Input: part model. Units: mm. Frame: model coordinates. Round coordinates to 2 decimals unless told otherwise and drop trailing zeros. Loops run counter-clockwise (first coordinate to the right, second up) from the corner with the lowest first, then second, coordinate; pieces in that order, holes last. Notation, with made-up numbers: (26.25, -16.5) - (62.25, -16.5) arc R32 cw to (62.25, 9.5) - close; hole circle Ø11 at (17.25, 4). An arc over 180 degrees is marked (long way). One line per question, with ' | ' between items. Start each with the question number.
Item 1: Section C-C, the plane z = 3.25. Return loops of the section in (x, y).
Item 2: Section B-B, the plane x = 10.25. Return loops of the section in (y, z).
Item 3: First-contact query: pin 1 (0.7 mm diameter, centred on y = 6.5, z = 4, fed in from +X); pin 2 (0.5 mm diameter, centred on x = 6.5, y = 5, fed in from +Z); pin 3 (0.5 mm diameter, centred on x = 14, y = 6.5, fed in from -Z). Flat tips, straight axial feed; report the tip coordinate or a pass-through.
Item 4: Section A-A, the plane y = 4.5. Give the number of separate pieces and of enclosed holes in the cut face, plus the area to 3 significant figures.
Item 5: Draft query along X for faces 1 (the face through (10, 1, 0)), 2 (the face through (0, 1, 3)), 3 (the face through (10, 2.5, 2)), 4 (the face through (20, 1, 3)). Return one class per face: pulls with the +X half, pulls with the -X half, needs draft (parallel to the pull), parting line crosses it, or undercut.
Item 6: Material intervals for line 1 along Z through (x, y) = (14, 5); line 2 along Y through (x, z) = (4.75, 3.5); line 3 along X through (y, z) = (1.75, 4.65), sorted ascending.
```python
from build123d import *

# Parameters (mm, degrees)
ESQUISSE1_W        = 20
ESQUISSE1_H        = 5
BOSS_EXTRU_1_DEPTH = 2.5
ESQUISSE2_W        = 0.6
ESQUISSE2_H        = 0.6
BOSS_EXTRU_2_DEPTH = 6
CHANFREIN1_SIZE    = 0.1
CHANFREIN2_SIZE    = 0.5


with BuildPart() as part:
    # Esquisse1 → Boss.-Extru.1 (new body)
    with BuildSketch(Plane(origin=(0, 0, 0), x_dir=(1, 0, 0), z_dir=(0, 1, 0))):
        with Locations((10, -2.5)):
            Rectangle(ESQUISSE1_W, ESQUISSE1_H)
    extrude(amount=BOSS_EXTRU_1_DEPTH)

    # Esquisse2 → Boss.-Extru.2 (add)
    with BuildSketch(Plane(origin=(0, 2.5, 0), x_dir=(1, 0, 0), z_dir=(0, 1, 0))):
        with Locations((1.1, -1.2)):
            Rectangle(ESQUISSE2_W, ESQUISSE2_H)
        with Locations((1.1, -3.74)):
            Rectangle(ESQUISSE2_W, ESQUISSE2_H)
        with Locations((3.64, -1.2)):
            Rectangle(ESQUISSE2_W, ESQUISSE2_H)
        with Locations((3.64, -3.74)):
            Rectangle(ESQUISSE2_W, ESQUISSE2_H)
        with Locations((6.18, -1.2)):
            Rectangle(ESQUISSE2_W, ESQUISSE2_H)
        with Locations((6.18, -3.74)):
            Rectangle(ESQUISSE2_W, ESQUISSE2_H)
        with Locations((8.72, -1.2)):
            Rectangle(ESQUISSE2_W, ESQUISSE2_H)
        with Locations((8.72, -3.74)):
            Rectangle(ESQUISSE2_W, ESQUISSE2_H)
        with Locations((11.26, -1.2)):
            Rectangle(ESQUISSE2_W, ESQUISSE2_H)
        with Locations((11.26, -3.74)):
            Rectangle(ESQUISSE2_W, ESQUISSE2_H)
        with Locations((13.8, -1.2)):
            Rectangle(ESQUISSE2_W, ESQUISSE2_H)
        with Locations((13.8, -3.74)):
            Rectangle(ESQUISSE2_W, ESQUISSE2_H)
        with Locations((16.34, -1.2)):
            Rectangle(ESQUISSE2_W, ESQUISSE2_H)
        with Locations((16.34, -3.74)):
            Rectangle(ESQUISSE2_W, ESQUISSE2_H)
        with Locations((18.88, -1.2)):
            Rectangle(ESQUISSE2_W, ESQUISSE2_H)
        with Locations((18.88, -3.74)):
            Rectangle(ESQUISSE2_W, ESQUISSE2_H)
    extrude(amount=BOSS_EXTRU_2_DEPTH)

    # Chanfrein1
    chanfrein1_edges = [part.edges().sort_by_distance(p)[0] for p in [
        (10.96, 8.5, 1.2),
        (11.26, 8.5, 1.5),
        (11.56, 8.5, 1.2),
        (11.26, 8.5, 0.9),
        (10.96, 8.5, 3.74),
        (11.26, 8.5, 4.04),
        (11.56, 8.5, 3.74),
        (11.26, 8.5, 3.44),
        (13.5, 8.5, 1.2),
        (13.8, 8.5, 1.5),
        (14.1, 8.5, 1.2),
        (13.8, 8.5, 0.9),
        (13.5, 8.5, 3.74),
        (13.8, 8.5, 4.04),
        (14.1, 8.5, 3.74),
        (13.8, 8.5, 3.44),
        (16.04, 8.5, 1.2),
        (16.34, 8.5, 1.5),
        (16.64, 8.5, 1.2),
        (16.34, 8.5, 0.9),
        (16.04, 8.5, 3.74),
        (16.34, 8.5, 4.04),
        (16.64, 8.5, 3.74),
        (16.34, 8.5, 3.44),
        (18.58, 8.5, 1.2),
        (18.88, 8.5, 1.5),
        (19.18, 8.5, 1.2),
        (0.8, 8.5, 1.2),
        (18.88, 8.5, 0.9),
        (1.1, 8.5, 1.5),
        (1.4, 8.5, 1.2),
        (1.1, 8.5, 0.9),
        (18.58, 8.5, 3.74),
        (18.88, 8.5, 4.04),
        (19.18, 8.5, 3.74),
        (18.88, 8.5, 3.44),
        (0.8, 8.5, 3.74),
        (1.1, 8.5, 4.04),
        (1.4, 8.5, 3.74),
        (1.1, 8.5, 3.44),
        (3.34, 8.5, 1.2),
        (3.64, 8.5, 1.5),
        (3.94, 8.5, 1.2),
        (3.64, 8.5, 0.9),
        (3.34, 8.5, 3.74),
        (3.64, 8.5, 4.04),
        (3.94, 8.5, 3.74),
        (3.64, 8.5, 3.44),
        (5.88, 8.5, 1.2),
        (6.18, 8.5, 1.5),
        (6.48, 8.5, 1.2),
        (6.18, 8.5, 0.9),
        (5.88, 8.5, 3.74),
        (6.18, 8.5, 4.04),
        (6.48, 8.5, 3.74),
        (6.18, 8.5, 3.44),
        (8.42, 8.5, 1.2),
        (8.72, 8.5, 1.5),
        (9.02, 8.5, 1.2),
        (8.72, 8.5, 0.9),
        (8.42, 8.5, 3.74),
        (8.72, 8.5, 4.04),
        (9.02, 8.5, 3.74),
        (8.72, 8.5, 3.44),
    ]]
    chamfer(chanfrein1_edges, length=CHANFREIN1_SIZE)

    # Chanfrein2
    chanfrein2_edges = [part.edges().sort_by_distance(p)[0] for p in [
        (0, 1.25, 0),
        (20, 1.25, 0),
        (20, 1.25, 5),
        (0, 1.25, 5),
    ]]
    chamfer(chanfrein2_edges, length=CHANFREIN2_SIZE)


solid = part.part
```
Return value:
1) outline: (0, 0) - (20, 0) - (20, 2.5) - (0, 2.5) - close
2) outline: (0, 0) - (2.5, 0) - (2.5, 5) - (0, 5) - close
3) pin 1: x = 19.18 | pin 2: z = 4.04 | pin 3: z = 0.9
4) separate pieces: 16 | enclosed holes: 0 | area: 5.76 mm2
5) face 1: needs draft | face 2: pulls with the -X half | face 3: undercut | face 4: pulls with the +X half
6) line 1: 0.9 to 1.5, 3.44 to 4.04 | line 2: 0 to 2.5 | line 3: 0.15 to 19.85
